from build123d import *

# Parameters (mm, degrees)
BOSS_EXTRUDE1_DEPTH                               = 3
CONVERT_SOLID1_DEPTH                              = 1
SKETCH8_R                                         = 2
CUT_EXTRUDE1_DEPTH                                = 2
CSK_FOR_4_FLAT_HEAD_MACHINE_SCREW_100_D           = 3.2639
CSK_FOR_4_FLAT_HEAD_MACHINE_SCREW_100_DEPTH       = 2
CSK_FOR_4_FLAT_HEAD_MACHINE_SCREW_100_CSINK_D     = 5.715
CSK_FOR_4_FLAT_HEAD_MACHINE_SCREW_100_CSINK_ANGLE = 100
CSK_FOR_4_FLAT_HEAD_MACHINE_SCREW_100_TIP         = 0.980574487


# Read off the part's stored shape, not the designer's step: Convert-Solid1
with BuildPart() as part:
    # Sketch2 → Boss-Extrude1 (new body)
    with BuildSketch(Plane(origin=(0, 0, 0), x_dir=(1, 0, 0), z_dir=(0, 1, 0))):
        with BuildLine():
            Line((-29.33, 9.113793118), (-29.33, 22.932784456))
            Line((-29.33, 22.932784456), (-29.33, 47.932784456))
            Line((-29.33, 47.932784456), (-19.33, 47.932784456))
            Line((-19.33, 47.932784456), (-19.33, 22.932784456))
            Line((-19.33, 22.932784456), (28.55, 22.932784456))
            Line((28.55, 22.932784456), (28.55, 9.612784456))
            ThreePointArc((28.55, 9.612784456), (22.487022583, 11.115362203), (16.57, 9.113793118))
            ThreePointArc((16.57, 9.113793118), (11.475, 7.507664738), (6.38, 9.113793118))
            ThreePointArc((6.38, 9.113793118), (0, 11.125), (-6.38, 9.113793118))
            ThreePointArc((-6.38, 9.113793118), (-11.475, 7.507664738), (-16.57, 9.113793118))
            ThreePointArc((-16.57, 9.113793118), (-22.95, 11.125), (-29.33, 9.113793118))
        make_face()
    extrude(amount=BOSS_EXTRUDE1_DEPTH)

    # Convert-Solid1 outline → Convert-Solid1 (cut)
    with BuildSketch(Plane(origin=(0, 0, 0), x_dir=(1, 0, 0), z_dir=(0, 1, 0))):
        with BuildLine():
            Line((-29.33, 47.932784456), (-29.33, 9.113793118))
            ThreePointArc((-29.33, 9.113793118), (-22.95, 11.125), (-16.57, 9.113793118))
            ThreePointArc((-16.57, 9.113793118), (-11.475, 7.507664738), (-6.38, 9.113793118))
            ThreePointArc((-6.38, 9.113793118), (0, 11.125), (6.38, 9.113793118))
            ThreePointArc((6.38, 9.113793118), (11.475, 7.507664738), (16.57, 9.113793118))
            ThreePointArc((16.57, 9.113793118), (22.487022583, 11.115362203), (28.55, 9.612784456))
            Line((28.55, 9.612784456), (28.55, 22.932784456))
            Line((28.55, 22.932784456), (-19.33, 22.932784456))
            Line((-19.33, 22.932784456), (-19.33, 47.932784456))
            Line((-19.33, 47.932784456), (-29.33, 47.932784456))
        make_face()
    extrude(amount=CONVERT_SOLID1_DEPTH, mode=Mode.SUBTRACT)

    # Sketch8 → Cut-Extrude1 (cut)
    with BuildSketch(Plane(origin=(0, 3, 0), x_dir=(1, 0, 0), z_dir=(0, 1, 0))):
        with Locations(Location((-24.33, 41.432784456, 0), (0, 0, 270))):
            Circle(SKETCH8_R)
        with Locations(Location((-24.33, 31.932784456, 0), (0, 0, 270))):
            Circle(SKETCH8_R)
    extrude(amount=-CUT_EXTRUDE1_DEPTH, mode=Mode.SUBTRACT)

    # CSK for #4 Flat Head Machine Screw (100)1
    with Locations(Plane(origin=(0, 3, 0), x_dir=(1, 0, 0), z_dir=(0, 1, 0))):
        with Locations((9.256666667, 16.762784456), (-10.036666667, 16.762784456)):
            CounterSinkHole(CSK_FOR_4_FLAT_HEAD_MACHINE_SCREW_100_D / 2, CSK_FOR_4_FLAT_HEAD_MACHINE_SCREW_100_CSINK_D / 2, depth=CSK_FOR_4_FLAT_HEAD_MACHINE_SCREW_100_DEPTH, counter_sink_angle=CSK_FOR_4_FLAT_HEAD_MACHINE_SCREW_100_CSINK_ANGLE)
            with Locations((0, 0, -(CSK_FOR_4_FLAT_HEAD_MACHINE_SCREW_100_DEPTH + CSK_FOR_4_FLAT_HEAD_MACHINE_SCREW_100_TIP / 2))):  # 118° drill point
                Cone(0, CSK_FOR_4_FLAT_HEAD_MACHINE_SCREW_100_D / 2, CSK_FOR_4_FLAT_HEAD_MACHINE_SCREW_100_TIP, mode=Mode.SUBTRACT)


solid = part.part
CAD build for the part. Positions are in the model's coordinates, mm. A direction names the side the tool comes from. Give positions to 0.01 mm unless a question says otherwise; leave off trailing zeros. Loops run counter-clockwise (first coordinate to the right, second up) from the corner with the lowest first, then second, coordinate; pieces in that order, holes last. Notation, with made-up numbers: M 26.5,-26 L 69.5,-26 A18 ccw 69.5,-10 Z; hole C -18,-7.5 d10. An arc over 180 degrees is marked long. One line per question, with ' | ' between items. Start each with the question number.
1. Two-plate mould, pull along Z, no slides. Class faces 1 (the face through (-22.64, 2.01, -30.86)), 2 (the face through (-23.729, 2.014, -39.525)), 3 (the face through (-29.33, 2, -28)), 4 (the face through (22.58, 1.99, -11.12)): pulls with the +Z half, pulls with the -Z half, needs draft (parallel to the pull), parting line crosses it, or undercut.
2. Probe L1, parallel to X at y = 1.3, z = -29; L2, parallel to Z at x = 11, y = 1.3; L3, parallel to Z at x = -24.5, y = 2.45. List the from-to ranges inside material, lowest first. Write a range as from..to.
3. Saw through at A-A on x = -25. Give the cut face in (y, z), plus the area to 3 significant figures.
4. Saw through at D-D on x = 14.5. Give the cut face in (y, z).
5. Saw through at C-C on z = -16. State how many separate pieces and enclosed holes the cut face has, plus the area to 3 significant figures.
6. Flat gauge pins, fed straight in: pin 1 (1 mm diameter, centred on y = 2.5, z = -30, fed in from +X); pin 2 (12 mm diameter, centred on x = 16.5, z = -29, fed in from -Y); pin 3 (4.5 mm diameter, centred on x = -24.33, z = -31.93, fed in from -Y); pin 4 (1 mm diameter, centred on x = -14.5, y = 1.5, fed in from -Z). Where does each tip first touch, or does it go through?
7. 3-axis set-ups, long thin cutter, end or side, ignore diameter. For faces 5 (the face through (4, 2, -22.933)), 6 (the face through (9.47, 1.48, -18.38)): which of +Z, -Z, +X, -X, +Y, -Y reach the whole face in a straight line?
8. Saw through at B-B on y = 1.4. Give the cut face in (x, z) (3 decimals), plus the area to 3 significant figures.
Result sheet:
1) face 1: undercut | face 2: undercut | face 3: needs draft | face 4: pulls with the +Z half
2) L1: x = -29.33..-19.33 | L2: z = -22.93..-7.52 | L3: z = -47.93..-43.43, -39.44..-33.93, -29.94..-11.02
3) outline: M 1,-47.93 L 3,-47.93 L 3,-43.32 L 1,-43.32 Z; M 1,-39.55 L 3,-39.55 L 3,-33.82 L 1,-33.82 Z; M 1,-30.05 L 3,-30.05 L 3,-10.93 L 1,-10.93 Z | area: 58.9 mm^2
4) outline: M 1,-22.93 L 3,-22.93 L 3,-8.04 L 1,-8.04 Z
5) separate pieces: 3 | enclosed holes: 0 | area: 101 mm^2
6) pin 1: stops at x = -19.33 | pin 2: passes through | pin 3: stops at y = 1 | pin 4: stops at z = -22.93
7) face 5: -Z, +X, +Y, -Y | face 6: +Y, -Y
8) outline: M -29.33,-47.933 L -19.33,-47.933 L -19.33,-22.933 L 28.55,-22.933 L 28.55,-9.613 A11.125 cw 16.57,-9.114 A8.884 ccw 6.38,-9.114 A11.125 cw -6.38,-9.114 A8.884 ccw -16.57,-9.114 A11.125 cw -29.33,-9.114 Z; hole C -24.33,-41.433 d4; hole C -24.33,-31.933 d4; hole C -10.037,-16.763 d3.264; hole C 9.257,-16.763 d3.264 | area: 978 mm^2
